The figure shows three views and two pictorial views of one solid part (mm, origin at its lowest corner). Answer the questions. Coordinates: 2 decimals unless noted, no trailing zeros. Write each loop counter-clockwise with the first axis right and the second up, starting at its lowest first coordinate (ties: lowest second). Pieces come first, ordered by that corner, then holes. Notation, with made-up numbers: (17, -2.5) -> (61, -2.5) arc R23 cw to (61, 26.5) -> close; hole circle Ø9 at (16.25, 34). An arc over 180 degrees is marked (long way). Use CSV: the item, a comma, the result in double quotes. Start each with the question number.
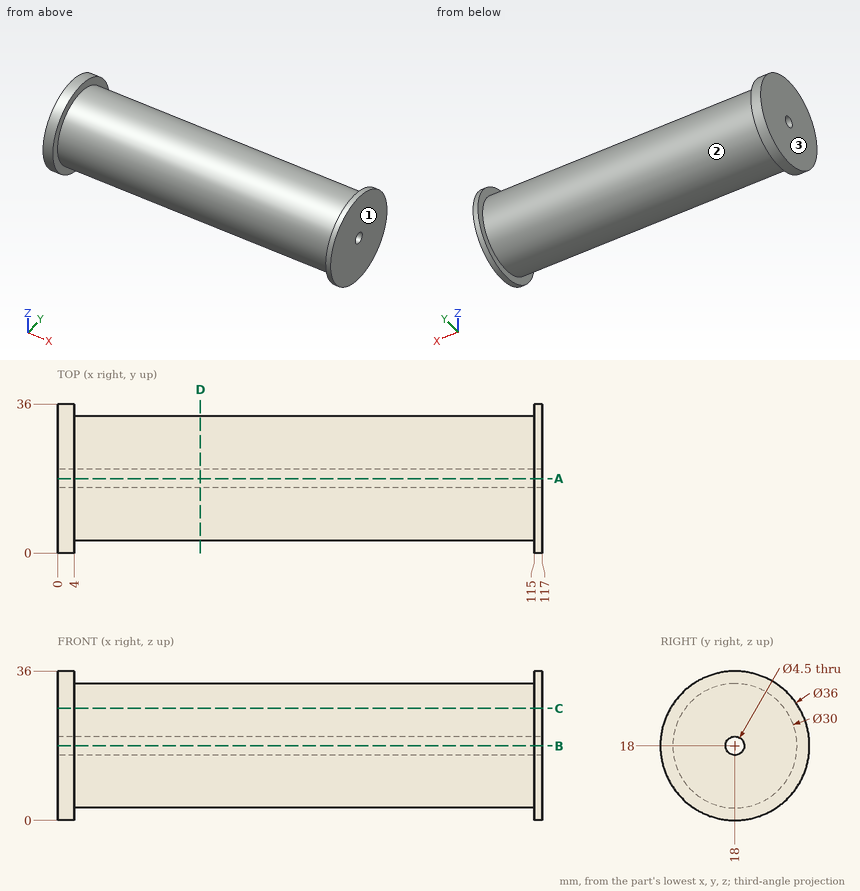
1) The mould has two halves that part along X. Classify the marked faces 1, 2 and 3: pulls with the +X half, pulls with the -X half, needs draft (parallel to the pull), parting line crosses it, or undercut.
2) Section A-A, the plane y = 18 is taken. Give the vertices of the cut face in (x, z).
3) Section C-C, the plane z = 27 is taken. Give the vertices of the cut face in (x, y).
4) Each of these flat-tipped pins is pushed along its axis until it touches: pin 1 (1.5 mm diameter, centred on y = 16.5, z = 14.5, fed in from -X); pin 2 (8 mm diameter, centred on x = 17, y = 23, fed in from -Z); pin 3 (3.5 mm diameter, centred on y = 18, z = 18, fed in from +X); pin 4 (10 mm diameter, centred on x = 76, z = 32.5, fed in from -Y). Where does it stop, or does it pass through?
5) Section D-D, the plane x = 34.5 is taken. Give the vertices of the cut face in (y, z), plus the area to 3 significant figures.
6) Find the intervals of material crossed by line 1 along Y through (x, z) = (28, 18); line 2 along Z through (x, y) = (53, 19.5); line 3 along Y through (x, z) = (91.5, 27), in increasing order.
The answers:
1,face 1,"pulls with the +X half"
1,face 2,"undercut"
1,face 3,"pulls with the -X half"
2,outline,"(0, 0) -> (4, 0) -> (4, 3) -> (115, 3) -> (115, 0) -> (117, 0) -> (117, 15.75) -> (0, 15.75) -> close; (0, 20.25) -> (117, 20.25) -> (117, 36) -> (115, 36) -> (115, 33) -> (4, 33) -> (4, 36) -> (0, 36) -> close"
3,outline,"(0, 2.41) -> (4, 2.41) -> (4, 6) -> (115, 6) -> (115, 2.41) -> (117, 2.41) -> (117, 33.59) -> (115, 33.59) -> (115, 30) -> (4, 30) -> (4, 33.59) -> (0, 33.59) -> close"
4,pin 1,"stops at x = 0"
4,pin 2,"stops at z = 3.03"
4,pin 3,"passes through"
4,pin 4,"stops at y = 6.39"
5,outline,"circle Ø30 at (18, 18); hole circle Ø4.5 at (18, 18)"
5,area,"691 mm^2"
6,line 1,"y = 3 to 15.75, 20.25 to 33"
6,line 2,"z = 3.08 to 16.32, 19.68 to 32.92"
6,line 3,"y = 6 to 30"
